Input: part model. Units: mm. Frame: model coordinates. Face numbers are marked on the shaded views. A direction names the side the tool comes from. Coordinates: 2 decimals unless noted, no trailing zeros. Order: outer loops, then holes, each group sorted by start corner. A loop starts at its lowest first (then second) coordinate and runs counter-clockwise, first axis right, second up. Notation, with made-up numbers: M -37,38 L 17,38 A25 cw 17,54 Z; hole C -38,-16 d3. An arc over 180 degrees is marked long. One line per item, written item: value.
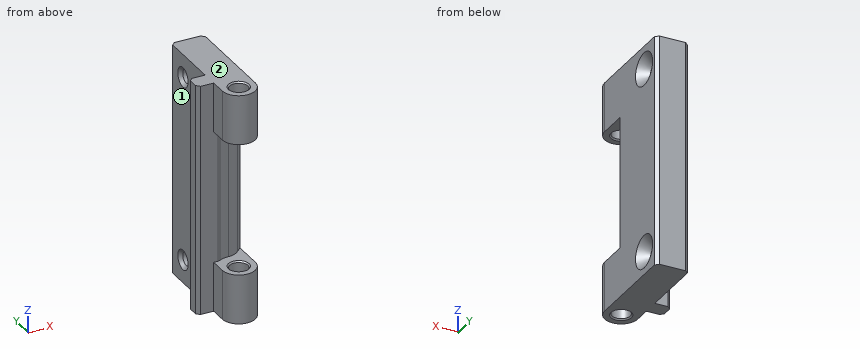
```python
from build123d import *

# Parameters (mm, degrees)
SKETCH007_R          = 2.75
PAD004_DEPTH         = 35
SKETCH008_W          = 10
SKETCH008_H          = 10
POCKET003_DEPTH      = 20
SKETCH009_R          = 6
POCKET004_DEPTH      = 20
CHAMFER007_SIZE      = 0.4
CHAMFER008_SIZE      = 0.4
CHAMFER009_SIZE      = 1
SKETCH014_R          = 2
POCKET008_DEPTH      = 10.001
POCKET008_DEPTH_BACK = 5.001
CHAMFER014_SIZE      = 1
CHAMFER019_SIZE      = 3
POCKET011_DEPTH      = 20
FILLET007_R          = 5


with BuildPart() as part:
    # Sketch007 → Pad004 (new body, symmetric)
    with BuildSketch(Plane.XY):
        with BuildLine():
            ThreePointArc((-5, 0), (0, -5), (5, 0))
            Line((5, 30), (5, 0))
            Line((-5, 30), (5, 30))
            Line((-5, 10), (-5, 30))
            Line((-10, 10), (-5, 10))
            Line((-10, 5), (-10, 10))
            Line((-5, 5), (-10, 5))
            Line((-5, 0), (-5, 5))
        make_face()
        Circle(SKETCH007_R, mode=Mode.SUBTRACT)
    extrude(amount=PAD004_DEPTH, both=True)

    # Sketch008 → Pocket003 (cut, symmetric)
    with BuildSketch(Plane.XY):
        Rectangle(SKETCH008_W, SKETCH008_H)
    extrude(amount=POCKET003_DEPTH, both=True, mode=Mode.SUBTRACT)

    # Sketch009 → Pocket004 (cut, symmetric)
    with BuildSketch(Plane.XY):
        Circle(SKETCH009_R)
    extrude(amount=POCKET004_DEPTH, both=True, mode=Mode.SUBTRACT)

    # Chamfer007
    chamfer007_edges = [part.edges().sort_by_distance(p)[0] for p in [
        (-3.316625, 5, 0),
    ]]
    chamfer(chamfer007_edges, length=CHAMFER007_SIZE)

    # Chamfer008
    chamfer008_edges = [part.edges().sort_by_distance(p)[0] for p in [
        (-2.75, 0, 20),
        (-2.75, 0, -20),
        (-2.75, 0, -35),
        (-2.75, 0, 35),
    ]]
    chamfer(chamfer008_edges, length=CHAMFER008_SIZE)

    # Chamfer009
    chamfer009_edges = [part.edges().sort_by_distance(p)[0] for p in [
        (-10, 5, 0),
        (-10, 10, 0),
        (5, 30, 0),
        (-5, 30, 0),
    ]]
    chamfer(chamfer009_edges, length=CHAMFER009_SIZE)

    # Sketch014 → Pocket008 (cut, two sides)
    with BuildSketch(Plane.YZ) as pocket008_sk:
        with Locations((23, 28)):
            Circle(SKETCH014_R)
        with Locations((23, -28)):
            Circle(SKETCH014_R)
    extrude(amount=-POCKET008_DEPTH, mode=Mode.SUBTRACT)
    extrude(pocket008_sk.sketch, amount=POCKET008_DEPTH_BACK, mode=Mode.SUBTRACT)

    # Chamfer014
    chamfer014_edges = [part.edges().sort_by_distance(p)[0] for p in [
        (-5, 21, -28),
        (-5, 21, 28),
    ]]
    chamfer(chamfer014_edges, length=CHAMFER014_SIZE)

    # Chamfer019
    chamfer019_edges = [part.edges().sort_by_distance(p)[0] for p in [
        (5, 21, 28),
        (5, 21, -28),
    ]]
    chamfer(chamfer019_edges, length=CHAMFER019_SIZE)

    # Sketch018 → Pocket011 (cut, symmetric)
    with BuildSketch(Plane.XY):
        Polygon((5, 9), (1, 5), (5, 5), align=None)
    extrude(amount=POCKET011_DEPTH, both=True, mode=Mode.SUBTRACT)

    # Fillet007
    fillet007_edges = [part.edges().sort_by_distance(p)[0] for p in [
        (1.741657, 5.741657, 0),
    ]]
    fillet(fillet007_edges, radius=FILLET007_R)


solid = part.part
```
(1) Access query for the marked faces 1 and 2. Directions: +Z, -Z, +X, -X, +Y, -Y. A direction counts if a zero-diameter tool reaches every point of the face in a straight line with its end or side. Return the directions, or none.
Data:
face 1: +Z, -Z, -X, +Y
face 2: +Z, +X, -X, +Y, -Y
(2) Cut plane D-D on z = 1.5. Output: boundary loops of the cut face in (x, y), plus the area to 3 significant figures.
Data:
outline: M -10,6 L -9,5 L -3.72,5 L -2.98,5.21 A6 cw -0.04,6 A5 ccw 3.46,7.46 L 5,9 L 5,29 L 4,30 L -4,30 L -5,29 L -5,10 L -9,10 L -10,9 Z
area: 261 mm2
(3) Cut plane A-A on y = 23. Output: boundary loops of the cut face in (x, z).
Data:
outline: M -5,-35 L 5,-35 L 5,-33 L 2,-30 L -4,-30 L -5,-31 Z; M -5,-25 L -4,-26 L 2,-26 L 5,-23 L 5,23 L 2,26 L -4,26 L -5,25 Z; M -5,31 L -4,30 L 2,30 L 5,33 L 5,35 L -5,35 Z
(4) First-contact query: pin 1 (1.6 mm diameter, centred on x = -7.5, z = -11.5, fed in from -Y); pin 2 (8 mm diameter, centred on y = 14.5, z = 18.5, fed in from -X). Flat tips, straight axial feed; report the tip coordinate or a pass-through.
Data:
pin 1: stops at y = 5
pin 2: stops at x = -5
(5) Cut plane C-C on y = 4. Output: boundary loops of the cut face in (x, z), plus the area to 3 significant figures.
Data:
outline: M -5,-35 L 5,-35 L 5,-20 L -5,-20 Z; M -5,20 L 5,20 L 5,35 L -5,35 Z
area: 300 mm2
(6) Ray query, line 1 (Z direction, x = -1.1, y = 23); line 2 (X direction, y = 0, z = 31.75); line 3 (Y direction, x = 0, z = -28). Return the intervals inside material, ascending. Write a range as from..to.
Data:
line 1: z = -35..-30, -26..26, 30..35
line 2: x = -5..-2.75, 2.75..5
line 3: y = -5..-2.75, 2.75..21, 25..30
(7) Cut plane B-B on z = 28. Output: boundary loops of the cut face in (x, y).
Data:
outline: M -10,6 L -9,5 L -5,5 L -5,0 A5 ccw 5,0 L 5,18 L 2,21 L -4,21 L -5,20 L -5,10 L -9,10 L -10,9 Z; M -5,26 L -4,25 L 2,25 L 5,28 L 5,29 L 4,30 L -4,30 L -5,29 Z; hole C 0,0 d5.5
